Autodesk Inventor part; units mm, degrees
ref_plane "工作平面1" through (-20, 0, 0) normal (0, -1, 0) x (1, 0, 0)
ref_plane "YZ Plane" through (0, 0, 0) normal (1, 0, 0) x (0, 1, 0)
ref_plane "XZ Plane" through (0, 0, 0) normal (0, 1, 0) x (-1, 0, 0)
sketch "草圖2" plane through (0, 0, 0) normal (0, 0, 1) x (1, 0, 0)
  arc A0 (12, 0) -> (-12, 0) centre (0, 0) ccw
  arc A1 (20, 0) -> (-20, 0) centre (0, 0) ccw
  line L0 (-20, 0) -> (-12, 0)
  line L1 (12, 0) -> (20, 0)
  dimension "d4" = 24
  dimension "d5" = 40
extrude "擠出1" add sketch "草圖2" along normal blind 130
ref_plane "工作平面1" through (-20, 0, 0) normal (0, -1, 0) x (1, 0, 0)
sketch "草圖3" plane through (-20, 0, 0) normal (0, -1, 0) x (1, 0, 0)
  line L0 (40, 130) -> (0, 130)
  line L1 (0, 130) -> (4, 130)
  line L2 (0, 0) -> (40, 0)
  line L3 (40, 0) -> (36, 0)
  circle A0 centre (4, 30) radius 1.4
  circle A1 centre (4, 100) radius 1.4
  circle A2 centre (36, 100) radius 1.4
  circle A3 centre (36, 30) radius 1.4
  point P0 (20, 0)
  dimension "d9" = 4
  dimension "d10" = 4
  dimension "d13" = 2.8
  dimension "d14" = 2.8
  dimension "d15" = 2.8
  dimension "d16" = 2.8
extrude "擠出2" cut sketch "草圖3" against normal blind 8
properties part number "holding_positionLFT"
Here's how the part is built. I have some questions about the finished solid (model axes, mm). A direction names the side the tool comes from. Round coordinates to 2 decimals unless told otherwise and drop trailing zeros. Write each loop counter-clockwise with the first axis right and the second up, starting at its lowest first coordinate (ties: lowest second). Pieces come first, ordered by that corner, then holes. Notation, with made-up numbers: (43, -8) -> (77, -8) arc R34 cw to (77, 26) -> close; hole circle Ø4 at (-38.75, 33). An arc over 180 degrees is marked (long way). One line per item, written item: value.
1) Suppose I cut it at B-B on x = 16. List the corners of the cut face in (y, z) for me.
Filled sheet:
outline: (0, 0) -> (12, 0) -> (12, 130) -> (0, 130) -> (0, 101.4) -> (8, 101.4) -> (8, 98.6) -> (0, 98.6) -> (0, 31.4) -> (8, 31.4) -> (8, 28.6) -> (0, 28.6) -> close
2) Suppose I cut it at C-C on z = 30. List the corners of the cut face in (x, y) for me.
Filled sheet:
outline: (-20, 0) -> (-17.4, 0) -> (-17.4, 8) -> (-14.6, 8) -> (-14.6, 0) -> (-12, 0) arc R12 cw to (12, 0) -> (14.6, 0) -> (14.6, 8) -> (17.4, 8) -> (17.4, 0) -> (20, 0) arc R20 ccw to start
3) Suppose I cut it at D-D on y = 16. List the corners of the cut face in (x, z) for me, plus the area to 3 significant figures.
Filled sheet:
outline: (-12, 0) -> (12, 0) -> (12, 130) -> (-12, 130) -> close
area: 3,120 mm2
4) I'm going to push flat-ended pins straight in: pin 1 Ø0.8 at (x, z) = (16.5, 30.5) entering from -Y; pin 2 Ø10 at (y, z) = (6, 48) entering from +X (3 decimals); pin 3 Ø3 at (y, z) = (5.5, 101.5) entering from +X. Where does each tip first touch, or does it pass through?
Filled sheet:
pin 1: stops at y = 8
pin 2: stops at x = 19.975
pin 3: stops at x = 19.6
5) Suppose I cut it at A-A on y = 6. List the corners of the cut face in (x, z) for me, plus the area to 3 significant figures.
Filled sheet:
outline: (-19.08, 0) -> (-10.39, 0) -> (-10.39, 130) -> (-19.08, 130) -> close; (10.39, 0) -> (19.08, 0) -> (19.08, 130) -> (10.39, 130) -> close; hole circle Ø2.8 at (-16, 30); hole circle Ø2.8 at (-16, 100); hole circle Ø2.8 at (16, 30); hole circle Ø2.8 at (16, 100)
area: 2,230 mm2
6) For faces 4 (the face through (16, 0, 64)), 5 (the face through (-16, 8, 30)), which set-ups out of +Z, -Z, +X, -X, +Y, -Y let a thin tool reach every point of the face, with its end or its side?
Filled sheet:
face 4: +Z, -Z, +X, -X, -Y
face 5: -Y
7) We'd pull the mould along Z, two halves only. Please class faces 1 (the face through (15.697, 3.944, 98.633)), 2 (the face through (-0.3, 12.4, 130)), 3 (the face through (-0.3, 12.4, 0)): released by +Z, released by -Z, zero draft, split by the parting line, or undercut.
Filled sheet:
face 1: undercut
face 2: released by +Z
face 3: released by -Z
8) If I drill on line 1 (Z direction, x = 16, y = 2.5); line 2 (X direction, y = 4, z = 100); line 3 (X direction, y = 3, z = 100), over which ranges is the centre line in solid material (lowest first)? Write a range as [from, to].
Filled sheet:
line 1: z = [0, 28.6], [31.4, 98.6], [101.4, 130]
line 2: x = [-19.6, -17.4], [-14.6, -11.31], [11.31, 14.6], [17.4, 19.6]
line 3: x = [-19.77, -17.4], [-14.6, -11.62], [11.62, 14.6], [17.4, 19.77]
